Autodesk Inventor part; units mm, degrees
ref_plane "YZ Plane" through (0, 0, 0) normal (1, 0, 0) x (0, 1, 0)
ref_plane "XZ Plane" through (0, 0, 0) normal (0, 1, 0) x (-1, 0, 0)
ref_plane "XY Plane" through (0, 0, 0) normal (0, 0, 1) x (1, 0, 0)
sketch "Sketch1" plane through (0, 0, 0) normal (0, 1, 0) x (-1, 0, 0)
  line L0 (0, 0) -> (125, 0)
  line L1 (125, 0) -> (125, 150)
  line L2 (125, 150) -> (0, 150)
  line L3 (0, 150) -> (0, 0)
  dimension "d0" = 125
  dimension "d1" = 150
extrude "Extrusion1" add sketch "Sketch1" along normal blind 10
sketch "Sketch2" plane through (0, 10, 0) normal (0, 1, 0) x (1, 0, 0)
  line L0 (-125, -150) -> (0, -150)
  line L1 (0, -150) -> (-4, -150)
  line L2 (-4, -150) -> (-4, -4)
  line L3 (-4, -4) -> (-125, -4)
  line L4 (-125, 0) -> (-125, -150)
  line L5 (0, -150) -> (0, 0)
  line L6 (0, 0) -> (-125, 0)
  line L7 (-125, 0) -> (-125, -150)
  line L8 (-125, -150) -> (0, -150)
  dimension "d4" = 4
  dimension "d5" = 146
extrude "Extrusion2" add sketch "Sketch2" along normal blind 125 contours L2 L3 L4 L6 L5 L0
sketch "Sketch4" plane through (-125, 10, 4) normal (0, 0, 1) x (1, 0, 0)
  line L0 (0, -10) -> (0, 0)
  line L1 (0, 0) -> (0, 20)
  line L2 (0, -10) -> (0, 125)
  line L3 (0, 20) -> (20, 20)
  line L4 (20, 20) -> (86, 20)
  line L5 (86, 20) -> (86, 47)
  line L6 (86, 47) -> (20, 47)
  line L7 (20, 47) -> (20, 20)
  line L8 (20, 47) -> (20, 67)
  line L9 (20, 67) -> (20, 90)
  line L10 (20, 90) -> (20, 67)
  line L11 (20, 67) -> (81.6, 67)
  point P0 (125, -10)
  point P1 (0, -5)
  dimension "d11" = 20
  dimension "d12" = 20
  dimension "d13" = 66
  dimension "d14" = 27
  dimension "d15" = 20
  dimension "d55" = 23
  dimension "d56" = 61.6
extrude "Extrusion4" cut sketch "Sketch4" against normal blind 10
sketch "Sketch7" plane through (-125, 0, 150) normal (0, 0, 1) x (1, 0, 0)
  line L0 (125, 0) -> (0, 0)
  line L1 (125, 0) -> (125, 5)
  line L2 (125, 0) -> (125, 135)
  line L3 (125, 5) -> (10, 5)
  line L4 (10, 5) -> (10, 0)
  line L5 (10, 0) -> (125, 0)
  dimension "d32" = 5
  dimension "d33" = 115
extrude "Extrusion6" cut sketch "Sketch7" against normal blind 20
sketch "Sketch9" plane through (0, 0, 0) normal (0, -1, 0) x (1, 0, 0)
  line L0 (0, 130) -> (-115, 130)
  line L1 (0, 130) -> (-65, 130)
  line L2 (-65, 130) -> (-65, 80)
  line L3 (-65, 80) -> (-45, 80)
  line L4 (-45, 80) -> (-85, 80)
  point P0 (0, 0)
  dimension "d40" = 65
  dimension "d41" = 50
  dimension "d42" = 20
  dimension "d43" = 40
hole "Hole2" at (-45, 0, 80) at (-85, 0, 80) direction (0, 1, 0) diameter 4 end through all counterbore diameter 6 counterbore depth 3
sketch "Sketch10" plane through (0, 135, 0) normal (0, 0, -1) x (-1, 0, 0)
  line L0 (0, 0) -> (125, 0)
  line L1 (125, 0) -> (125, -10)
  line L2 (125, -125) -> (125, 0)
  line L3 (125, -10) -> (4, -10)
  line L4 (4, -125) -> (4, 0)
  line L5 (4, -10) -> (4, -15)
  line L6 (4, -15) -> (125, -15)
  line L7 (125, -15) -> (125, -10)
  line L8 (125, -16.3986) -> (125, -10)
  line L9 (125, -10) -> (125, -15)
  point P0 (0, -135)
  dimension "d51" = 10
  dimension "d52" = 5
extrude "Extrusion8" cut sketch "Sketch10" against normal blind 10 contours L3 L2 L6 L4
hole "Hole3" at (-105, 100, 4) at (-43.4, 77, 4) direction (0, 0, -1) diameter 3.5 end through all
sketch "Sketch12" plane through (-125, 0, 0) normal (-1, 0, 0) x (0, 0, 1)
  line L0 (150, 0) -> (140, 0)
  line L1 (140, 0) -> (140, 5)
  line L2 (150, 5) -> (130, 5)
  line L3 (140, 5) -> (0, 5)
  line L4 (0, 0) -> (0, 120)
  line L5 (0, 0) -> (0, 5)
  line L6 (4, 120) -> (0, 120)
  line L7 (0, 0) -> (0, 120)
  line L8 (0, 0) -> (150, 0)
  line L9 (150, 0) -> (150, 10)
  line L10 (4, 10) -> (150, 10)
  line L11 (4, 10) -> (4, 120)
  dimension "d77" = 10
extrude "Extrusion9" add sketch "Sketch12" along normal blind 20 contours L8 L4 L3 L2 L1
sketch "Sketch11" plane through (0, 10, 0) normal (0, 1, 0) x (1, 0, 0)
  line L0 (-115, -150) -> (-115, -130)
  line L1 (-115, -150) -> (-78, -150)
  line L2 (-125, -150) -> (-4, -150)
  line L3 (-78, -150) -> (-78, -140)
  line L4 (-78, -140) -> (-41, -140)
  line L5 (-125, -140) -> (-125, -150)
  line L6 (-125, -140) -> (-125, -94.6667)
  line L7 (-125, -4) -> (-125, -150)
  line L8 (-125, -94.6667) -> (-135, -94.6667)
  line L9 (-135, -94.6667) -> (-135, -49.3333)
  point P0 (0, 0)
  dimension "d67" = 37
  dimension "d68" = 10
  dimension "d69" = 37
  dimension "d80" = 45.3333
  dimension "d81" = 45.3333
hole "Hole4" at (-78, 10, 140) at (-41, 10, 140) direction (0, -1, 0) diameter 4.318 end through all
hole "Hole5" at (-135, 10, 94.6667) at (-135, 10, 49.3333) direction (0, -1, 0) diameter 3.5 end through all
sketch "Sketch13" plane through (0, 0, 0) normal (0, -1, 0) x (1, 0, 0)
  circle A0 centre (-135, 94.6667) radius 1.75
  circle A1 centre (-135, 49.3333) radius 1.75
  circle A2 centre (-45, 80) radius 3
  circle A3 centre (-85, 80) radius 3
  line L0 (0, 130) -> (-115, 130)
  line L1 (-115, 130) -> (-115, 150)
  line L2 (-125, 150) -> (-115, 150)
  line L3 (-125, 140) -> (-125, 150)
  line L4 (-125, 140) -> (-145, 140)
  line L5 (-145, 0) -> (-145, 140)
  line L6 (0, 0) -> (-145, 0)
  line L7 (0, 130) -> (0, 0)
extrude "Extrusion10" add sketch "Sketch13" along normal blind 3
sketch "Sketch14" plane through (-45, 3, 80) normal (0, -1, 0) x (1, 0, 0)
  circle A0 centre (0, 0) radius 3
  circle A1 centre (0, 0) radius 2
  circle A2 centre (-40, 0) radius 3
  circle A3 centre (-40, 0) radius 2
  point P0 (45, -80)
extrude "Extrusion11" add sketch "Sketch14" along normal blind 3
sketch "Sketch15" plane through (0, -3, 0) normal (0, -1, 0) x (1, 0, 0)
  circle A0 centre (-135, 49.3333) radius 1.75
  circle A1 centre (-135, 94.6667) radius 1.75
  point P0 (0, 0)
hole "Hole6" at (-135, -3, 94.6667) at (-135, -3, 49.3333) direction (0, 1, 0) diameter 4.318 end through all counterbore diameter 7.62 counterbore depth 5.08
properties part number "Quarter 3"
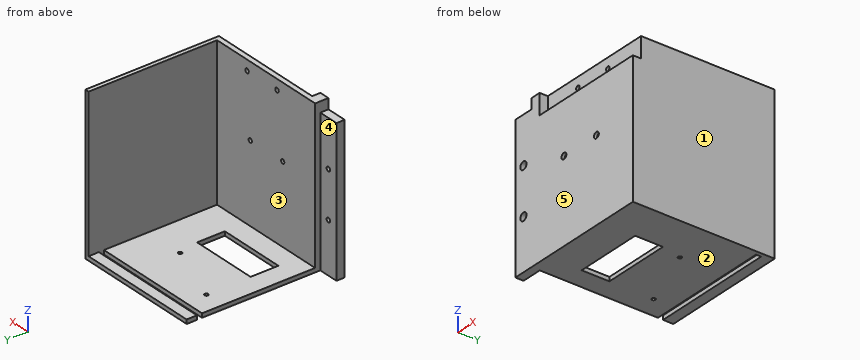
Source: CAD feature listing. Evaluate the final solid. Frame: model axes, mm. Face numbers are marked on the shaded views. A direction names the side the tool comes from. Coordinates: 2 decimals unless noted, no trailing zeros. Loops run counter-clockwise (first coordinate to the right, second up) from the corner with the lowest first, then second, coordinate; pieces in that order, holes last. Notation, with made-up numbers: M -36,-35.75 L 6,-35.75 A20 ccw 6,-12.75 Z; hole C 74.5,37.25 d2. An arc over 180 degrees is marked long. Answer in a Markdown table with one row per item.
Q1. Ray query, probe 1 along Z at (x, y) = (-135, -0.9); probe 2 along X at (y, z) = (6.75, 80); probe 3 along X at (y, z) = (8.05, 140). Return the intervals inside material, ascending. Write a range as from..to.
Answers below:
| item | result |
|---|---|
| probe 1 | z = 0..45.52, 53.14..90.86, 98.48..140 |
| probe 2 | x = -125..-87, -83..-47, -43..0 |
| probe 3 | x = -125..-80.16, -75.84..-43.16, -38.84..0 |
Q2. Section B-B on y = 46. Return the cut outline in (x, z), plus the area to 3 significant figures.
Answers below:
| item | result |
|---|---|
| outline | M -125,0 L -105,0 L -105,4 L -125,4 Z; M -39,0 L 0,0 L 0,150 L -4,150 L -4,4 L -39,4 Z |
| area | 820 mm^2 |
Q3. Section A-A on x = -135. Return the cut outline in (y, z).
Answers below:
| item | result |
|---|---|
| outline | M -3,0 L 5,0 L 5,47.17 L 2.08,47.17 L 2.08,45.52 L -3,45.52 Z; M -3,53.14 L 2.08,53.14 L 2.08,51.49 L 5,51.49 L 5,92.51 L 2.08,92.51 L 2.08,90.86 L -3,90.86 Z; M -3,98.48 L 2.08,98.48 L 2.08,96.83 L 5,96.83 L 5,140 L -3,140 Z |
Q4. Section D-D on z = 55.5. Return the cut outline in (x, y), plus the area to 4 significant figures.
Answers below:
| item | result |
|---|---|
| outline | M -145,-3 L 0,-3 L 0,135 L -4,135 L -4,10 L -125,10 L -125,5 L -145,5 Z |
| area | 2,285 mm^2 |
Q5. First-contact query: pin 1 (3.5 mm diameter, centred on x = -41, z = 140, fed in from +Y); pin 2 (4.5 mm diameter, centred on y = 132, z = 2.5, fed in from -X); pin 3 (10 mm diameter, centred on x = -75.5, y = 111, fed in from +Z); pin 4 (10 mm diameter, centred on x = -140, z = 97.5, fed in from +Y). Flat tips, straight axial feed; report the tip coordinate or a pass-through.
Answers below:
| item | result |
|---|---|
| pin 1 | passes through |
| pin 2 | stops at x = -125 |
| pin 3 | stops at z = 4 |
| pin 4 | stops at y = 5 |
Q6. Draft query along X for the marked faces 1 and 2. Return one class per face: pulls with the +X half, pulls with the -X half, needs draft (parallel to the pull), parting line crosses it, or undercut.
Answers below:
| item | result |
|---|---|
| face 1 | pulls with the +X half |
| face 2 | needs draft |
Q7. Set-up query: the marked faces 3, 4 and 5. Return all of +Z, -Z, +X, -X, +Y, -Y with unobstructed straight access to the full face (end or side cutting, diameter ignored); none if empty.
Answers below:
| item | result |
|---|---|
| face 3 | +Z, -X, +Y |
| face 4 | +Z, -Z, -X, +Y |
| face 5 | +Z, -Z, +X, -X, -Y |
Q8. Section C-C on x = -31.5. Return the cut outline in (y, z).
Answers below:
| item | result |
|---|---|
| outline | M -3,0 L 120,0 L 120,4 L 10,4 L 10,150 L 5,150 L 5,130 L -3,130 Z; M 125,0 L 135,0 L 135,4 L 125,4 Z |
